Design review of the part shown in the three views and the two pictorial views. Dimensions are in mm from the part's minimum x, y and z. Give positions to 0.01 mm unless a question says otherwise; leave off trailing zeros. Loops run counter-clockwise (first coordinate to the right, second up) from the corner with the lowest first, then second, coordinate; pieces in that order, holes last. Notation, with made-up numbers: (19, 61.25) -> (59, 61.25) arc R7 ccw to (59, 70.25) -> close; hole circle Ø8 at (44, 76.25). An arc over 180 degrees is marked (long way). Answer as CSV lines item,"result".
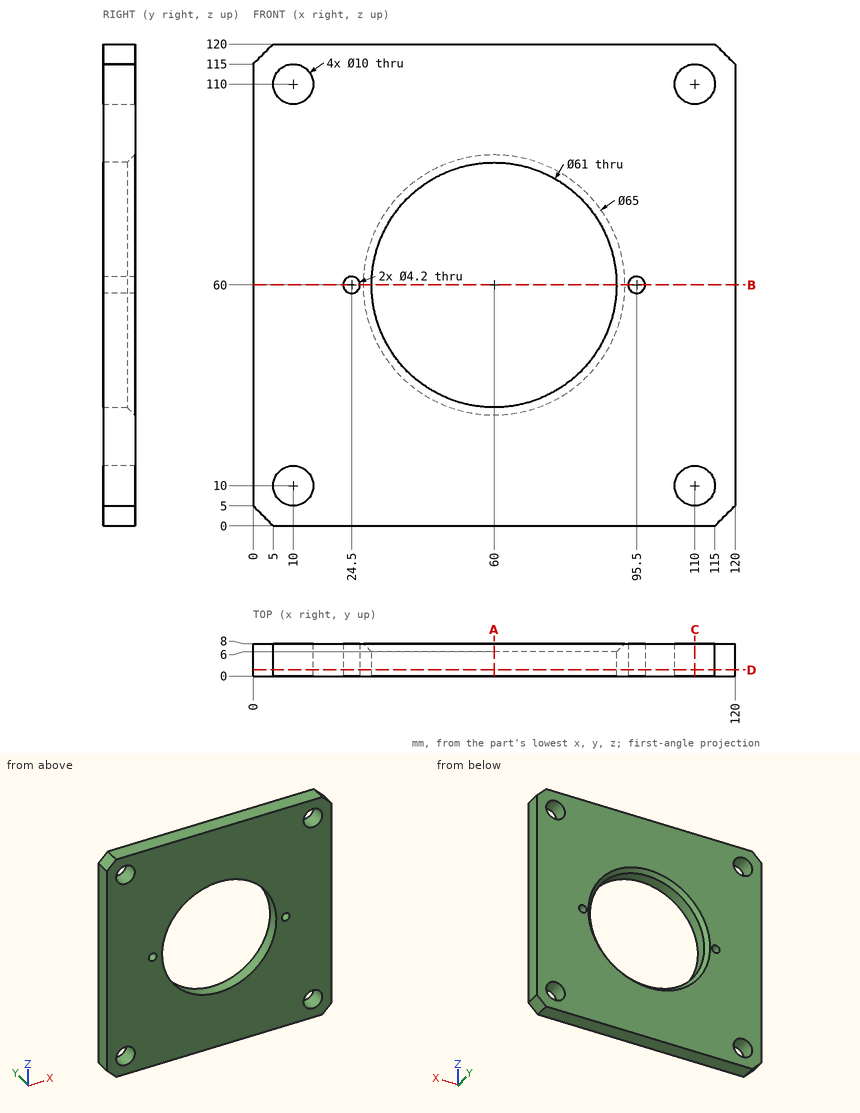
Q1. We need section D-D, the plane y = 1.5. State the section outline as (x, z) points, and give its area (3 significant figures).
Filled sheet:
outline,"(0, 5) -> (5, 0) -> (115, 0) -> (120, 5) -> (120, 115) -> (115, 120) -> (5, 120) -> (0, 115) -> close; hole circle Ø10 at (10, 10); hole circle Ø10 at (10, 110); hole circle Ø4.2 at (24.5, 60); hole circle Ø61 at (60, 60); hole circle Ø4.2 at (95.5, 60); hole circle Ø10 at (110, 10); hole circle Ø10 at (110, 110)"
area,"11,100 mm^2"
Q2. We need section A-A, the plane x = 60. State the section outline as (y, z) points, and give its area (3 significant figures).
Filled sheet:
outline,"(0, 0) -> (8, 0) -> (8, 27.5) -> (6, 29.5) -> (0, 29.5) -> close; (0, 90.5) -> (6, 90.5) -> (8, 92.5) -> (8, 120) -> (0, 120) -> close"
area,"468 mm^2"
Q3. We need section C-C, the plane x = 110. State the section outline as (y, z) points, and give its area (3 significant figures).
Filled sheet:
outline,"(0, 0) -> (8, 0) -> (8, 5) -> (0, 5) -> close; (0, 15) -> (8, 15) -> (8, 105) -> (0, 105) -> close; (0, 115) -> (8, 115) -> (8, 120) -> (0, 120) -> close"
area,"800 mm^2"
Q4. We need section B-B, the plane z = 60. State the section outline as (x, y) points.
Filled sheet:
outline,"(0, 0) -> (22.4, 0) -> (22.4, 8) -> (0, 8) -> close; (26.6, 0) -> (29.5, 0) -> (29.5, 6) -> (27.5, 8) -> (26.6, 8) -> close; (90.5, 0) -> (93.4, 0) -> (93.4, 8) -> (92.5, 8) -> (90.5, 6) -> close; (97.6, 0) -> (120, 0) -> (120, 8) -> (97.6, 8) -> close"
Q5. To check wall thickness, follow probe 1 along X at (y, z) = (3.25, 110); probe 2 along X at (y, z) = (7, 58.5); probe 3 along Z at (x, y) = (24.5, 4.5). State the ranges of each line that lie inside material, in increasing order. Write a range as from..to.
Filled sheet:
probe 1,"x = 0..5, 15..105, 115..120"
probe 2,"x = 0..23.03, 25.97..28.54, 91.46..94.03, 96.97..120"
probe 3,"z = 0..57.9, 62.1..120"
